The model under review builds one solid part; all positions refer to its coordinate system, in mm. Face numbers are marked on the shaded views. Round coordinates to 2 decimals unless told otherwise and drop trailing zeros. Order: outer loops, then holes, each group sorted by start corner. A loop starts at its lowest first (then second) coordinate and runs counter-clockwise, first axis right, second up.
1) Mouldability with a two-part tool opening along X and no side actions: class the marked faces 1, 2, 3 and 4 as pulls with the +X half, pulls with the -X half, needs draft (parallel to the pull), parting line crosses it, or undercut.
2) To check wall thickness, follow L1, parallel to Y at x = -5, z = 1.6; L2, parallel to X at y = 105.8, z = 8.25 (3 decimals); L3, parallel to Y at x = 94.1, z = 7. State the ranges of each line that lie inside material, in increasing order.
3) Consider section B-B (x = 61). Give the boundary of the cut face in (y, z), then the cut area to 3 significant figures.
4) Clearance check with flat-ended pins moving along their axes: P1, Ø2, axis at x = -5, y = 105.8, coming from the +Z side; P2, Ø11, axis at x = 67, y = 103.5, coming from the +Z side. State where each tip first meets the part, or that it passes through.
5) Consider section A-A (y = 10). Give the boundary of the cut face in (x, z), then the cut area to 3 significant figures.
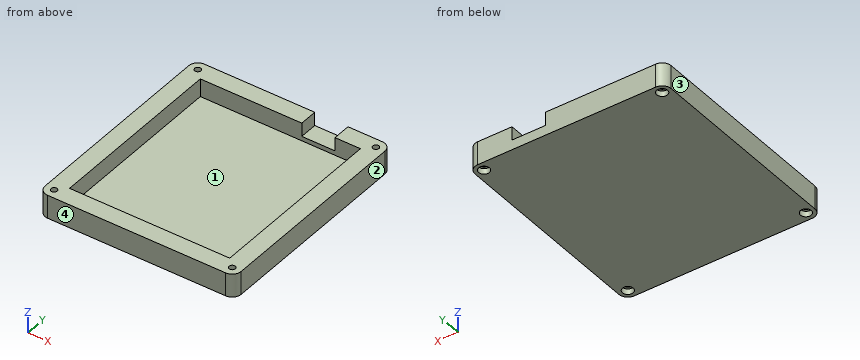
Autodesk Fusion 360 part; units mm, degrees
sketch "Schizzo1" plane through (0, 0, 0) normal (0, 0, 1) x (1, 0, 0)
  line L0 (0, 0) -> (89.1, 0)
  line L1 (89.1, 0) -> (89.1, 100.8)
  line L2 (89.1, 100.8) -> (0, 100.8)
  line L3 (0, 100.8) -> (0, 0)
  line L4 (-10, -10) -> (99.1, -10)
  line L5 (99.1, -10) -> (99.1, 110.8)
  line L6 (99.1, 110.8) -> (-10, 110.8)
  line L7 (-10, 110.8) -> (-10, -10)
  circle A0 centre (94.1, 105.8) radius 1.7
  circle A1 centre (94.1, 105.8) radius 3
  circle A2 centre (94.1, -5) radius 1.7
  circle A3 centre (94.1, -5) radius 3
  circle A4 centre (-5, -5) radius 1.7
  circle A5 centre (-5, -5) radius 3
  circle A6 centre (-5, 105.8) radius 1.7
  circle A7 centre (-5, 105.8) radius 3
  dimension "d5" = 10
  dimension "d6" = 10
  dimension "d7" = 109.1
  dimension "d8" = 89.1
  dimension "d9" = 100.8
  dimension "d10" = 120.8
  dimension "d11" = 3.4
  dimension "d14" = 6
  dimension "d15" = 3.4
  dimension "d18" = 5
  dimension "d19" = 5
  dimension "d20" = 5
  dimension "d21" = 5
  dimension "d22" = 6
  dimension "d23" = 3.4
  dimension "d24" = 5
  dimension "d25" = 5
  dimension "d26" = 6
  dimension "d27" = 3.4
  dimension "d28" = 5
  dimension "d29" = 5
  dimension "d30" = 6
extrude "Estrusione1" add sketch "Schizzo1" along normal blind 9.9 from surface at 3.1 contours A1 | A3 | A5 | A7 makes body 1 at (94.9125, -2.1121, 9.7) makes body 2 at (-2.0037, -5.1495, 9.7) makes body 3 at (92.0053, 103.6524, 9.7) makes body 4 at (-2.1809, 104.7739, 9.7)
extrude "Estrusione2" add sketch "Schizzo1" along normal blind 13 contours L4 L5 L6 L7 bodies 1 2 3 4
extrude "Estrusione3" add sketch "Schizzo1" along normal blind 3 contours L0 L1 L2 L3 bodies 1
sketch "Schizzo2" plane through (0, 0, 13) normal (0, 0, 1) x (-1, 0, 0)
  circle A0 centre (-94.1, 5) radius 1.7
  circle A1 centre (5, -105.8) radius 1.7
  line L0 (0, 0) -> (0, -100.8)
  line L1 (0, -100.8) -> (-89.1, -100.8)
  line L2 (-89.1, -100.8) -> (-89.1, 0)
  line L3 (-89.1, 0) -> (0, 0)
  line L4 (10, -110.8) -> (10, 10)
  line L5 (10, 10) -> (-99.1, 10)
  line L6 (-99.1, 10) -> (-99.1, -110.8)
  line L7 (-99.1, -110.8) -> (10, -110.8)
  circle A2 centre (5, 5) radius 1.7
  circle A3 centre (-94.1, -105.8) radius 1.7
  line L8 (-56.455, -110.8) -> (-74.955, -110.8)
  line L9 (-74.955, -110.8) -> (-74.955, -100.8)
  line L10 (-74.955, -100.8) -> (-56.455, -100.8)
  line L11 (-56.455, -100.8) -> (-56.455, -110.8)
  line L12 (10, -110.8) -> (10, 10)
  dimension "d38" = 18.5
  dimension "d39" = 66.455
extrude "Estrusione4" cut sketch "Schizzo2" against normal blind 7.5 contours L1 L7 L8 L9 L10 L11 bodies 1
fillet "Raccordo1" radius 5 4 edges at (99.1, -10, 6.5) (-10, -10, 6.5) (99.1, 110.8, 6.5) (-10, 110.8, 6.5) on bodies 1
Answer below:
1. face 1: undercut
1. face 2: pulls with the +X half
1. face 3: pulls with the -X half
1. face 4: needs draft
2. L1: y = -10 to -8, -2 to 102.8, 108.8 to 110.8
2. L2: x = -10 to -6.7, -3.3 to 56.455, 74.955 to 92.4, 95.8 to 99.1
2. L3: y = -10 to -6.7, -3.3 to 104.1, 107.5 to 110.8
3. outline: (-10, 0) - (110.8, 0) - (110.8, 5.5) - (100.8, 5.5) - (100.8, 3) - (0, 3) - (0, 13) - (-10, 13) - close
3. area: 487 mm2
4. P1: passes through
4. P2: stops at z = 5.5
5. outline: (-10, 0) - (99.1, 0) - (99.1, 13) - (89.1, 13) - (89.1, 3) - (0, 3) - (0, 13) - (-10, 13) - close
5. area: 527 mm2
